Can you work these out from the model? Positions are in its coordinate system, mm. A direction names the side the tool comes from. Round coordinates to 2 decimals unless told otherwise and drop trailing zeros. Order: outer loops, then holes, each group sorted by start corner. A loop starts at its lowest first (then second) coordinate and runs counter-clockwise, first axis right, second up. Notation, with made-up numbers: (52.5, 56.5) -> (63.5, 56.5) arc R28 ccw to (63.5, 77.5) -> close; hole circle Ø1 at (24.5, -17.5). An arc over 180 degrees is marked (long way). Use a Markdown table: item, result. Add a question column.
Q1. We'd pull the mould along Z, two halves only. Please class faces 1 (the face through (-46, 1, 17.884)), 2 (the face through (40.3, 1.4, -13.3)), 3 (the face through (43, 1, 23)): +Z half, -Z half, draft (parallel to the pull), parting line (faces both ways), or undercut.
Q2. If we section it at D-D on z = -28: List the corners of the cut face in (x, y) for me, plus the area to 3 significant figures.
Q3. I'm going to push flat-ended pins straight in: pin 1 Ø3 at (x, z) = (39.5, -12) entering from -Y; pin 2 Ø2 at (y, z) = (1, 38) entering from +X; pin 3 Ø3 at (x, z) = (46.5, 14.38) entering from +Y; pin 4 Ø1.2 at (y, z) = (2, 23.5) entering from +X. Where does each tip first touch, or does it pass through?
Q4. If we section it at B-B on x = 0: List the corners of the cut face in (y, z) for me, plus the area to 3 significant figures.
Q5. If we section it at A-A on x = -46.5: List the corners of the cut face in (y, z) for me.
Q6. I need wall thicknesses on line 1 along X through (y, z) = (2.25, -21); line 2 along X through (y, z) = (0.2, -21); line 3 along Z through (x, y) = (39, 0.25). Which ranges of each line are inside material? Lowest first, please. Write a range as [from, to].
Q7. If we section it at C-C on z = 14: List the corners of the cut face in (x, y) for me.
Q8. For faces 4 (the face through (-43, 1, 24)), 5 (the face through (-49.574, 0.217, 14.788)), 6 (the face through (37, 1, 30.766)), which set-ups out of +Z, -Z, +X, -X, +Y, -Y let a thin tool reach every point of the face, with its end or its side?
Autodesk Inventor part; units mm, degrees
ref_plane "YZ Plane" through (0, 0, 0) normal (1, 0, 0) x (0, 1, 0)
ref_plane "XZ Plane" through (0, 0, 0) normal (0, 1, 0) x (-1, 0, 0)
ref_plane "XY Plane" through (0, 0, 0) normal (0, 0, 1) x (1, 0, 0)
sketch "Szkic1" plane through (0, 0, 0) normal (0, 1, 0) x (-1, 0, 0)
  line L0 (50, 50) -> (-50, 50)
  line L1 (-50, 50) -> (-50, -50)
  line L2 (-50, -50) -> (50, -50)
  line L3 (50, -50) -> (50, 50)
  line L4 (50, 50) -> (-50, -50) construction
  line L5 (-50, 50) -> (50, -50) construction
  point P0 (0, 0)
  dimension "d0" = 100
  dimension "d1" = 100
extrude "Wyciągnięcie proste1" add sketch "Szkic1" along normal blind 3
sketch "Szkic2" plane through (0, 3, 0) normal (0, 1, 0) x (1, 0, 0)
  line L0 (50, -50) -> (50, 50)
  line L1 (50, 50) -> (-50, 50)
  line L2 (-50, 50) -> (-50, -50)
  line L3 (-50, -50) -> (50, -50)
  line L4 (-50, 50) -> (-19, 50)
  line L5 (-19, 50) -> (-19, 17)
  line L6 (-19, 17) -> (-50, 17)
  line L7 (-50, 17) -> (-50, 50)
  line L8 (50, 50) -> (19, 50)
  line L9 (19, 50) -> (19, 17)
  line L10 (19, 17) -> (50, 17)
  line L11 (50, 17) -> (50, 50)
  point P0 (0, 0)
  dimension "d4" = 31
  dimension "d5" = 33
  dimension "d6" = 31
extrude "Wyciągnięcie proste2" cut sketch "Szkic2" against normal through all contours L10 L9 L1 L0 | L2 L1 L5 L6
sketch "Szkic3" plane through (0, 3, 0) normal (0, 1, 0) x (1, 0, 0)
  line L0 (19, 17) -> (19, 50)
  line L1 (19, 50) -> (-19, 50)
  line L2 (-19, 50) -> (-19, 17)
  line L3 (-19, 17) -> (-50, 17)
  line L4 (-50, 17) -> (-50, -50)
  line L5 (-50, -50) -> (50, -50)
  line L6 (50, -50) -> (50, 17)
  line L7 (50, 17) -> (19, 17)
  line L8 (19, 50) -> (-19, 50)
  line L9 (-19, 50) -> (-19, 44)
  line L10 (-19, 44) -> (19, 44)
  line L11 (19, 44) -> (19, 50)
  point P0 (0, 0)
  dimension "d9" = 6
extrude "Wyciągnięcie proste3" cut sketch "Szkic3" against normal through all contours L10 L2 L1 L0
sketch "Szkic5" plane through (-50, 0, 50) normal (-1, 0, 0) x (0, 0, 1)
  line L0 (0, 0) -> (0, 3)
  line L1 (-67, 3) -> (-67, 0)
  line L2 (-67, 0) -> (0, 0)
  line L3 (0, 0) -> (0, 3)
  line L4 (-67, 3) -> (0, 3)
  line L5 (-4.6672, -3.25) -> (-21.0795, 10.5216)
  point P0 (-50, 0)
  point P1 (-12.1156, 3)
  point P2 (-8.5404, 0)
extrude "Wyciągnięcie proste5" cut sketch "Szkic5" against normal through all contours L2 L5 L4 L0
sketch "Szkic6" plane through (0, 0, 0) normal (0, -1, 0) x (1, 0, 0)
  line L0 (-50, 17.8844) -> (-43, 17.8844)
  line L1 (-50, 17.8844) -> (-43, 17.8844)
  line L2 (-43, 17.8844) -> (-43, 43.0531)
  line L3 (-43, 43.0531) -> (-50, 43.0531)
  line L4 (-50, 43.0531) -> (-50, 17.8844)
  point P0 (0, 0)
extrude "Wyciągnięcie proste6" cut sketch "Szkic6" against normal through all
ref_plane "Płaszczyzna konstrukcyjna1" through (0, 0, -17) normal (-1, 0, 0) x (0, 0, 1)
mirror "Odbij1" about plane through (0, 0, -17) normal (-1, 0, 0) of "Wyciągnięcie proste6"
sketch "Szkic8" plane through (0, 0, 0) normal (0, -1, 0) x (1, 0, 0)
  line L0 (50, 17.8844) -> (43, 17.8844)
  line L1 (43, 17.8844) -> (43, 41.4596)
  line L2 (43, 41.4596) -> (-43, 41.4596)
  line L3 (-43, 41.4596) -> (-43, 17.8844)
  line L4 (-43, 17.8844) -> (-50, 17.8844)
  line L5 (-50, -17) -> (-50, 17.8844)
  line L6 (-50, -17) -> (-19, -17)
  line L7 (-19, -17) -> (-19, -44)
  line L8 (-19, -44) -> (19, -44)
  line L9 (19, -44) -> (19, -17)
  line L10 (19, -17) -> (50, -17)
  line L11 (50, 17.8844) -> (50, -17)
  point P0 (0, 0)
extrude "Wyciągnięcie proste7" add sketch "Szkic8" along normal blind 1
sketch "Szkic9" plane through (-19, 3, -44) normal (-1, 0, 0) x (0, 0, 1)
  circle A0 centre (10, 9.75) radius 16
  circle A1 centre (10, 9.75) radius 14.5
  line L0 (0, 0) -> (0, -4)
  line L1 (27, -4) -> (0, -4)
  line L2 (27, 0) -> (27, -4)
  line L3 (0, 0) -> (27, 0)
  point P0 (44, -3)
  point P1 (5.397, -4)
  point P2 (0, -0.75)
  dimension "d21" = 1.5
extrude "Wyciągnięcie proste8" cut sketch "Szkic9" against normal through all contours L0 A1 L1 A0 | A0 L1 L0
sketch "Szkic10" plane through (0, -1, 0) normal (0, -1, 0) x (1, 0, 0)
  point P0 (0, 0)
sketch "Szkic11" plane through (0, -1, 0) normal (0, -1, 0) x (1, 0, 0)
  circle A0 centre (0, -39.5) radius 1.7
  circle A1 centre (-9, -21) radius 1.7
  circle A2 centre (9, -21) radius 1.7
  arc A3 (46.5, -10) -> (43, -13.5) centre (46.5, -13.5) ccw
  arc A4 (43, 14.3844) -> (47, 10.9203) centre (46.5, 14.3844) ccw
  arc A5 (-43, -13.5) -> (-46.5, -10) centre (-46.5, -13.5) ccw
  arc A6 (-47, 10.9203) -> (-43, 14.3844) centre (-46.5, 14.3844) ccw
  circle A7 centre (-39, -12) radius 1.55
  circle A8 centre (39, -12) radius 1.55
  point P0 (0, 0)
hole "Otwór1" at (-39, -1, -12) at (-46.5, -1, -13.5) at (-46.5, -1, 14.3844) at (-9, -1, -21) at (0, -1, -39.5) at (9, -1, -21) at (39, -1, -12) at (46.5, -1, -13.5) at (46.5, -1, 14.3844) direction (0, 1, 0) diameter 3.3 end through all counterbore diameter 6.2 counterbore depth 2.4
sketch "Szkic12" plane through (0, -1, 0) normal (0, -1, 0) x (1, 0, 0)
  arc A0 (2.9674, -38.603) -> (-2.9674, -38.603) centre (0, -39.5) ccw
  line L0 (2.9674, -38.603) -> (19, -38.603)
  line L1 (19, -38.603) -> (19, -17)
  line L2 (19, -17) -> (50, -17)
  line L3 (50, -17) -> (50, 17.8844)
  line L4 (50, 17.8844) -> (43, 17.8844)
  line L5 (43, 17.8844) -> (43, 41.4596)
  line L6 (43, 41.4596) -> (-43, 41.4596)
  line L7 (-43, 41.4596) -> (-43, 17.8844)
  line L8 (-43, 17.8844) -> (-50, 17.8844)
  line L9 (-50, 17.8844) -> (-50, -17)
  line L10 (-50, -17) -> (-19, -17)
  line L11 (-19, -17) -> (-19, -38.603)
  line L12 (-19, -38.603) -> (-2.9674, -38.603)
  circle A1 centre (46.5, 14.3844) radius 3.1
  circle A2 centre (39, -12) radius 3.1
  circle A3 centre (-46.5, 14.3844) radius 3.1
  circle A4 centre (-39, -12) radius 3.1
  circle A5 centre (-46.5, -13.5) radius 3.1
  circle A6 centre (-9, -21) radius 3.1
  circle A7 centre (9, -21) radius 3.1
  circle A8 centre (46.5, -13.5) radius 3.1
  line L13 (-50, 30.7663) -> (-50, 40.7446)
  line L14 (-43, 30.7663) -> (-50, 30.7663)
  line L15 (-43, 40.7446) -> (-43, 30.7663)
  line L16 (-43, 40.7446) -> (-50, 40.7446)
  line L17 (-50, 30.7663) -> (-30, 30.7663)
  line L18 (-30, 30.7663) -> (-30, 41.4596)
  line L19 (-30, 41.4596) -> (-50, 41.4596)
  line L20 (-50, 41.4596) -> (-50, 30.7663)
  line L21 (50, 30.7663) -> (50, 40.7446)
  line L22 (43, 40.7446) -> (50, 40.7446)
  line L23 (43, 40.7446) -> (43, 30.7663)
  line L24 (43, 30.7663) -> (50, 30.7663)
  line L25 (50, 30.7663) -> (30, 30.7663)
  line L26 (30, 30.7663) -> (30, 41.4596)
  line L27 (30, 41.4596) -> (50, 41.4596)
  line L28 (50, 41.4596) -> (50, 30.7663)
  circle A9 centre (46.1444, 33.7663) radius 1.1
  circle A10 centre (-46.1444, 33.7663) radius 1.1
  point P0 (0, 0)
  dimension "d31" = 20
  dimension "d32" = 20
extrude "Wyciągnięcie proste9" cut sketch "Szkic12" against normal through all contours L25 L26 L6 L5 | L5 L22 L21 L24 | L14 L13 L16 L7 | L7 L6 L18 L17 | L5 L27 L28 L22 | L16 L20 L19 L7 | A9 | A10
fillet "Zaokrąglenie2" radius 1.5 10 edges at (-50, 1, 17.8844) (-50, 1, -17) (-19, 1, -17) (19, 1, -17) (50, 1, -17) (50, 1, 17.8844) (43, 1, 30.7663) (30, 1, 30.7663) (-43, 1, 30.7663) (-30, 1, 30.7663)
properties part number "podstawa_kopia" material "Stal, odlew"
Answer below:
| question | item | result |
|---|---|---|
| 1 | face 1 | +Z half |
| 1 | face 2 | undercut |
| 1 | face 3 | draft |
| 2 | outline | (-19, -1) -> (19, -1) -> (19, 3) -> (-19, 3) -> close |
| 2 | area | 152 mm² |
| 3 | pin 1 | y = 1.4 |
| 3 | pin 2 | x = 30 |
| 3 | pin 3 | through |
| 3 | pin 4 | x = 43 |
| 4 | outline | (-1, -36.4) -> (1.4, -36.4) -> (1.4, -37.85) -> (3, -37.85) -> (3, 37.88) -> (0, 41.46) -> (-1, 41.46) -> close; (1.08, -42.6) arc R14.5 ccw to (2.25, -44) -> (3, -44) -> (3, -41.15) -> (1.4, -41.15) -> (1.4, -42.6) -> close |
| 4 | area | 313 mm² |
| 5 | outline | (-1, -17) -> (3, -17) -> (3, -15.15) -> (1.4, -15.15) -> (1.4, -16.6) -> (-1, -16.6) -> close; (-1, -10.4) -> (1.4, -10.4) -> (1.4, -11.85) -> (3, -11.85) -> (3, 12.73) -> (1.4, 12.73) -> (1.4, 11.28) -> (-1, 11.28) -> close; (-1, 17.48) -> (1.4, 17.48) -> (1.4, 16.03) -> (3, 16.03) -> (3, 17.88) -> (-1, 17.88) -> close |
| 6 | line 1 | [-19, -10.65], [-7.35, 7.35], [10.65, 19] |
| 6 | line 2 | [-19, -12.1], [-5.9, 5.9], [12.1, 19] |
| 6 | line 3 | [-17, -15.1], [-8.9, 30.77] |
| 7 | outline | (-50, -1) -> (-49.58, -1) -> (-49.58, 1.4) -> (-48.1, 1.4) -> (-48.1, 3) -> (-50, 3) -> close; (-44.9, 1.4) -> (-43.42, 1.4) -> (-43.42, -1) -> (43.42, -1) -> (43.42, 1.4) -> (44.9, 1.4) -> (44.9, 3) -> (-44.9, 3) -> close; (48.1, 1.4) -> (49.58, 1.4) -> (49.58, -1) -> (50, -1) -> (50, 3) -> (48.1, 3) -> close |
| 8 | face 4 | +Z, -X, +Y, -Y |
| 8 | face 5 | -Y |
| 8 | face 6 | +Z, +X, +Y, -Y |
